from build123d import *

# Parameters (mm, degrees)
SKETCH1_W           = 88.323262869
SKETCH1_H           = 29.809101218
BOSS_EXTRUDE1_DEPTH = 10
SKETCH2_W           = 13.924014339
SKETCH2_H           = 29.809101218
BOSS_EXTRUDE2_DEPTH = 20
RIB1_REACH          = 96.478
SKETCH4_WALL_W      = 235.275808006
SKETCH4_WALL_H      = 2
SKETCH5_R           = 5.326775894
SKETCH5_R_2         = 8.926735981
BOSS_EXTRUDE3_DEPTH = 20
RIB2_REACH          = 96.478
SKETCH6_WALL_W      = 222.44376487
SKETCH6_WALL_H      = 2
RIB2_DRAFT_ANGLE    = 4


with BuildPart() as part:
    # Sketch1 → Boss-Extrude1 (new body)
    with BuildSketch(Plane(origin=(0, 0, 0), x_dir=(1, 0, 0), z_dir=(0, 1, 0))):
        with Locations((44.161631435, -14.904550609)):
            Rectangle(SKETCH1_W, SKETCH1_H)
    extrude(amount=BOSS_EXTRUDE1_DEPTH)

    # Sketch2 → Boss-Extrude2 (add)
    with BuildSketch(Plane(origin=(0, 10, 0), x_dir=(1, 0, 0), z_dir=(0, 1, 0))):
        with Locations((41.809601986, -14.904550609)):
            Rectangle(SKETCH2_W, SKETCH2_H)
    extrude(amount=BOSS_EXTRUDE2_DEPTH)

    # Sketch4 wall → Rib1 (add, up to next)
    with BuildSketch(Plane(origin=(68.547436012, 20, 15), x_dir=(0.892394851297, -0.451255392631, 0), z_dir=(0.451255392631, 0.892394851297, 0)), mode=Mode.PRIVATE) as rib1_sk1:
        Rectangle(SKETCH4_WALL_W, SKETCH4_WALL_H)
    rib1_tool1 = extrude(rib1_sk1.sketch, amount=-RIB1_REACH, mode=Mode.PRIVATE) - part.part
    add(rib1_tool1.solids().sort_by_distance((68.547436012, 20, 15))[0])

    # Sketch5 → Boss-Extrude3 (add)
    with BuildSketch(Plane.XZ):
        with Locations(Location((20.255604114, 15, 0), (0, 0, 90))):
            Circle(SKETCH5_R)
        with Locations(Location((65.99787284, 15, 0), (0, 0, 90))):
            Circle(SKETCH5_R_2)
    extrude(amount=BOSS_EXTRUDE3_DEPTH)

    # Sketch6 wall → Rib2 (add, up to next)
    with BuildSketch(Plane(origin=(41.326758433, -20, 15), x_dir=(1, 0, 0), z_dir=(0, 1, 0)), mode=Mode.PRIVATE) as rib2_sk1:
        Rectangle(SKETCH6_WALL_W, SKETCH6_WALL_H)
    rib2_tool1 = extrude(rib2_sk1.sketch, amount=RIB2_REACH, mode=Mode.PRIVATE) - part.part
    add(rib2_tool1.solids().sort_by_distance((41.326758433, -20, 15))[0])

    # Rib2 draft
    rib2_draft_faces = [part.faces().sort_by_distance(p)[0] for p in [
        (41.326758433, -19.5, 14),
        (41.326758433, -19.5, 16),
    ]]
    draft(rib2_draft_faces, Plane(origin=(41.326758433, -20, 15), x_dir=(1, 0, 0), z_dir=(0, -1, 0)), RIB2_DRAFT_ANGLE)


solid = part.part
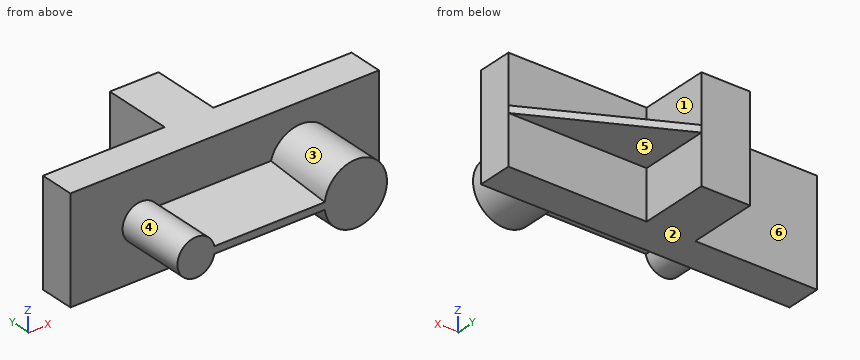
Geometry check sheet. Reference: the model listing, model coordinates, mm. Face numbers are marked on the shaded views. A direction names the side the tool comes from. Round coordinates to 2 decimals unless told otherwise and drop trailing zeros. Write each loop counter-clockwise with the first axis right and the second up, starting at its lowest first coordinate (ties: lowest second). Pieces come first, ordered by that corner, then holes. Notation, with made-up numbers: (22, 81.5) - (55, 81.5) arc R9 cw to (55, 91.5) - close; hole circle Ø1 at (34.5, -29.5). An arc over 180 degrees is marked (long way). One line per item, written item: value.
1. Mould release check, pull along X, two halves, no side actions. Record for the marked faces 1, 2 and 3: released by +X, released by -X, zero draft, split by the parting line, or undercut.
The answers:
face 1: released by +X
face 2: zero draft
face 3: undercut
2. Cross-section at A-A on z = 25. Record the boundary of the cut face in (x, y), and give its area (3 significant figures).
The answers:
outline: (0, 0) - (88.32, 0) - (88.32, 10) - (48.77, 10) - (48.77, 30) - (34.85, 30) - (34.85, 10) - (0, 10) - close
area: 1,160 mm^2
3. Cross-section at D-D on y = -2. Record the boundary of the cut face in (x, z), and give its area (3 significant figures).
The answers:
outline: (25.08, 12.74) - (57.36, 12.74) arc R8.93 ccw (long way) to (57.36, 17.26) - (25.08, 17.26) arc R5.33 ccw (long way) to start
area: 483 mm^2
4. Cross-section at C-C on z = 15. Record the boundary of the cut face in (x, y), and give its area (3 significant figures).
The answers:
outline: (0, 0) - (14.93, 0) - (14.93, -20) - (74.92, -20) - (74.92, 0) - (88.32, 0) - (88.32, 10) - (48.77, 30) - (34.85, 30) - (34.85, 10) - (0, 10) - close
area: 2,760 mm^2
5. Depth check by flat-ended pin: pin 1 Ø1.5 at (x, z) = (13, 18) entering from -Y; pin 2 Ø4 at (x, y) = (19, -7.5) entering from -Z; pin 3 Ø5 at (y, z) = (15.5, 3) entering from -X. Enter the tip coordinate at first touch or a pass-through.
The answers:
pin 1: stops at y = 0
pin 2: stops at z = 9.67
pin 3: stops at x = 34.85
6. Scan lines: L1, parallel to Y at x = 79, z = 2; L2, parallel to X at y = 28.5, z = 20.25; L3, parallel to X at y = -4.5, z = 10.5. Record each from-to range of solid material in increasing order.
The answers:
L1: y = 0 to 10
L2: x = 34.85 to 48.77
L3: x = 17.41 to 23.11, 58.29 to 73.71
7. Set-up check for the marked faces 4, 5 and 6: record each of +Z, -Z, +X, -X, +Y, -Y from which the full face is reachable in a straight line by a thin tool's end or side.
The answers:
face 4: -Y
face 5: -Z, +X, +Y
face 6: +Z, -Z, -X, +Y
8. Cross-section at B-B on x = 44. Record the boundary of the cut face in (y, z).
The answers:
outline: (-20, 14) - (0, 12.6) - (0, 0) - (30, 0) - (30, 29.81) - (0, 29.81) - (0, 17.4) - (-20, 16) - close
